Verification items for the finished model (mm, model axes). Face numbers are marked on the shaded views. A direction names the side the tool comes from. Coordinates: 2 decimals unless noted, no trailing zeros. Order: outer loops, then holes, each group sorted by start corner. A loop starts at its lowest first (then second) coordinate and runs counter-clockwise, first axis right, second up. Notation, with made-up numbers: (5.5, 6.5) - (54.5, 6.5) arc R26 cw to (54.5, 38.5) - close; hole circle Ø4 at (71.5, -14.75). An arc over 180 degrees is marked (long way). One line per question, with ' | ' between items. Start each with the question number.
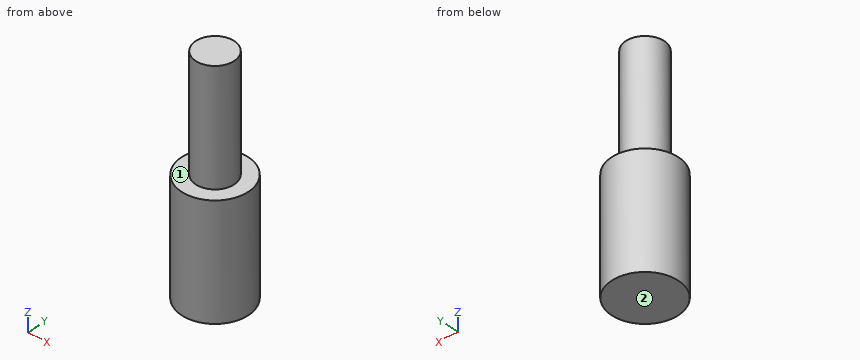
from build123d import *

# Parameters (mm, degrees)
CYLINDER1036_R     = 2.95
CYLINDER1036_DEPTH = 10
CYLINDER1037_R     = 1.7
CYLINDER1037_DEPTH = 10


with BuildPart() as cylinder1078:
    # Cylinder1036 → Cylinder1036 (new body)
    with BuildSketch(Plane.XY):
        Circle(CYLINDER1036_R)
    extrude(amount=CYLINDER1036_DEPTH)


with BuildPart() as m3boltshort:
    # Cylinder1037 → Cylinder1037 (new body)
    with BuildSketch(Plane.XY.offset(10)):
        Circle(CYLINDER1037_R)
    extrude(amount=CYLINDER1037_DEPTH)

    # Fusion114: union Cylinder1078
    add(cylinder1078.part)


solid = m3boltshort.part
Item 1: Gauge pin test, flat ends, axial feed: pin 1 (1.5 mm diameter, centred on x = -2, z = 7.5, fed in from +Y); pin 2 (1.5 mm diameter, centred on x = 1, y = -1.5, fed in from +Z); pin 3 (1 mm diameter, centred on y = -1.5, z = 17, fed in from +X); pin 4 (1.5 mm diameter, centred on y = -0.5, z = 16, fed in from +X). Record the tip position at first contact, or that the pin passes through.
Item 2: Section check D-D (x = -2.3). Record the cut outline in (y, z).
Item 3: Set-up check for the marked faces 1 and 2: record each of +Z, -Z, +X, -X, +Y, -Y from which the full face is reachable in a straight line by a thin tool's end or side.
Item 4: Section check C-C (z = 10.5). Record the cut outline in (x, y), then the cut area to 3 significant figures.
Item 5: Section check A-A (y = 0). Record the cut outline in (x, z).
Item 6: Thickness scan on probe 1 along Z at (x, y) = (-1.65, 2.4); probe 2 along X at (y, z) = (0.05, 18.75); probe 3 along X at (y, z) = (-0.2, 2.25). Record the ranges inside material, lowest first. Write a range as from..to.
Completed:
1) pin 1: stops at y = 2.67 | pin 2: stops at z = 20 | pin 3: stops at x = 1.37 | pin 4: stops at x = 1.7
2) outline: (-1.85, 0) - (1.85, 0) - (1.85, 10) - (-1.85, 10) - close
3) face 1: +Z | face 2: -Z, +X, -X, +Y, -Y
4) outline: circle Ø3.4 at (0, 0) | area: 9.08 mm^2
5) outline: (-2.95, 0) - (2.95, 0) - (2.95, 10) - (1.7, 10) - (1.7, 20) - (-1.7, 20) - (-1.7, 10) - (-2.95, 10) - close
6) probe 1: z = 0..10 | probe 2: x = -1.7..1.7 | probe 3: x = -2.94..2.94
